Check sheet for the modelled part. Datum: model origin and axes. Units: mm. Round coordinates to 2 decimals unless told otherwise and drop trailing zeros. Write each loop counter-clockwise with the first axis right and the second up, starting at its lowest first coordinate (ties: lowest second). Pieces come first, ordered by that corner, then holes. Notation, with made-up numbers: (-10.75, 88.25) -> (26.25, 88.25) arc R11 ccw to (26.25, 104.25) -> close; hole circle Ø1 at (-38, 67.25). An arc over 180 degrees is marked (long way). One line per item, written item: value.
from build123d import *

# Parameters (mm, degrees)
SKETCH1_W           = 18.54
SKETCH1_H           = 43.2
BOSS_EXTRUDE1_DEPTH = 1.5
SKETCH2_R           = 0.846666667
SKETCH2_R_2         = 0.423333333
CUT_EXTRUDE1_DEPTH  = 2.5


with BuildPart() as part:
    # Sketch1 → Boss-Extrude1 (new body)
    with BuildSketch(Plane(origin=(0, 0, 0), x_dir=(1, 0, 0), z_dir=(0, 1, 0))):
        Rectangle(SKETCH1_W, SKETCH1_H)
    extrude(amount=BOSS_EXTRUDE1_DEPTH)

    # Sketch2 → Cut-Extrude1 (cut, through all)
    with BuildSketch(Plane(origin=(0, 1.5, 0), x_dir=(1, 0, 0), z_dir=(0, 1, 0))):
        with Locations((7.9375, 20.32)):
            Circle(SKETCH2_R)
        with Locations((7.9375, -20.32)):
            Circle(SKETCH2_R)
        with Locations((-7.9375, -20.32)):
            Circle(SKETCH2_R)
        with Locations((-7.9375, 20.32)):
            Circle(SKETCH2_R)
        with Locations((-7.9375, -17.78)):
            Circle(SKETCH2_R_2)
        with Locations((-7.9375, -15.24)):
            Circle(SKETCH2_R_2)
        with Locations((-7.9375, -12.7)):
            Circle(SKETCH2_R_2)
        with Locations((-7.9375, -10.16)):
            Circle(SKETCH2_R_2)
        with Locations((-7.9375, -7.62)):
            Circle(SKETCH2_R_2)
        with Locations((-7.9375, -5.08)):
            Circle(SKETCH2_R_2)
        with Locations((-7.9375, -2.54)):
            Circle(SKETCH2_R_2)
        with Locations((-7.9375, 0)):
            Circle(SKETCH2_R_2)
        with Locations((-7.9375, 2.54)):
            Circle(SKETCH2_R_2)
        with Locations((-7.9375, 5.08)):
            Circle(SKETCH2_R_2)
        with Locations((-7.9375, 7.62)):
            Circle(SKETCH2_R_2)
        with Locations((-7.9375, 10.16)):
            Circle(SKETCH2_R_2)
        with Locations((-7.9375, 12.7)):
            Circle(SKETCH2_R_2)
        with Locations((-7.9375, 15.24)):
            Circle(SKETCH2_R_2)
        with Locations((-7.9375, 17.78)):
            Circle(SKETCH2_R_2)
        with Locations((7.9425, -15.24)):
            Circle(SKETCH2_R_2)
        with Locations((7.9425, -12.7)):
            Circle(SKETCH2_R_2)
        with Locations((7.9425, -10.16)):
            Circle(SKETCH2_R_2)
        with Locations((7.9425, -7.62)):
            Circle(SKETCH2_R_2)
        with Locations((7.9425, -5.08)):
            Circle(SKETCH2_R_2)
        with Locations((7.9425, -2.54)):
            Circle(SKETCH2_R_2)
        with Locations((7.9425, 0)):
            Circle(SKETCH2_R_2)
        with Locations((7.9425, 2.54)):
            Circle(SKETCH2_R_2)
        with Locations((7.9425, 5.08)):
            Circle(SKETCH2_R_2)
        with Locations((7.9425, 7.62)):
            Circle(SKETCH2_R_2)
        with Locations((7.9425, 10.16)):
            Circle(SKETCH2_R_2)
        with Locations((7.9425, 12.7)):
            Circle(SKETCH2_R_2)
        with Locations((7.9425, 15.24)):
            Circle(SKETCH2_R_2)
        with Locations((7.9425, 17.78)):
            Circle(SKETCH2_R_2)
        with Locations((7.9425, -17.78)):
            Circle(SKETCH2_R_2)
        with Locations((0, 20.32)):
            Circle(SKETCH2_R_2)
        with Locations((-2.54, 20.32)):
            Circle(SKETCH2_R_2)
        with Locations((2.54, 20.32)):
            Circle(SKETCH2_R_2)
        with Locations((-2.54, 17.78)):
            Circle(SKETCH2_R_2)
        with Locations((0, 17.78)):
            Circle(SKETCH2_R_2)
        with Locations((2.54, 17.78)):
            Circle(SKETCH2_R_2)
    extrude(amount=-CUT_EXTRUDE1_DEPTH, mode=Mode.SUBTRACT)


solid = part.part
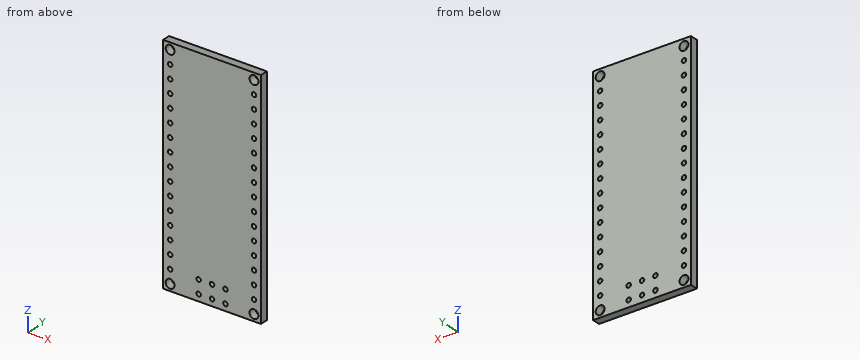
Item 1: Material ranges on line 1 along X through (y, z) = (1.05, 5.08); line 2 along Z through (x, y) = (0, 1.2); line 3 along Z through (x, y) = (-7.25, 1), recorded low to high.
Result set:
line 1: -9.27 to -8.36, -7.51 to 7.52, 8.37 to 9.27
line 2: -21.6 to -20.74, -19.9 to -18.2, -17.36 to 21.6
line 3: -21.6 to -20.81, -19.83 to 19.83, 20.81 to 21.6
Item 2: Depth check by flat-ended pin: pin 1 (1.5 mm diameter, centred on x = 7.94, z = 20.32, fed in from +Y); pin 2 (4 mm diameter, centred on x = 0, z = -1, fed in from -Y). Enter the tip coordinate at first touch or a pass-through.
Result set:
pin 1: through
pin 2: y = 0
Item 3: Sectioned sample at A-A (z = 15.24). Enter the section's corners in (x, y), then the cut area to 3 significant figures.
Result set:
outline: (-9.27, 0) -> (-8.36, 0) -> (-8.36, 1.5) -> (-9.27, 1.5) -> close; (-7.51, 0) -> (7.52, 0) -> (7.52, 1.5) -> (-7.51, 1.5) -> close; (8.37, 0) -> (9.27, 0) -> (9.27, 1.5) -> (8.37, 1.5) -> close
area: 25.3 mm^2
Item 4: Sectioned sample at C-C (z = -17.78). Enter the section's corners in (x, y).
Result set:
outline: (-9.27, 0) -> (-8.36, 0) -> (-8.36, 1.5) -> (-9.27, 1.5) -> close; (-7.51, 0) -> (-2.96, 0) -> (-2.96, 1.5) -> (-7.51, 1.5) -> close; (-2.12, 0) -> (-0.42, 0) -> (-0.42, 1.5) -> (-2.12, 1.5) -> close; (0.42, 0) -> (2.12, 0) -> (2.12, 1.5) -> (0.42, 1.5) -> close; (2.96, 0) -> (7.52, 0) -> (7.52, 1.5) -> (2.96, 1.5) -> close; (8.37, 0) -> (9.27, 0) -> (9.27, 1.5) -> (8.37, 1.5) -> close
Item 5: Sectioned sample at D-D (y = 0.25). State how many separate pieces and enclosed holes the cut face has, then the cut area to 3 significant figures.
Result set:
separate pieces: 1
enclosed holes: 40
area: 772 mm^2
Item 6: Sectioned sample at B-B (x = 0). Enter the section's corners in (y, z).
Result set:
outline: (0, -21.6) -> (1.5, -21.6) -> (1.5, -20.74) -> (0, -20.74) -> close; (0, -19.9) -> (1.5, -19.9) -> (1.5, -18.2) -> (0, -18.2) -> close; (0, -17.36) -> (1.5, -17.36) -> (1.5, 21.6) -> (0, 21.6) -> close
